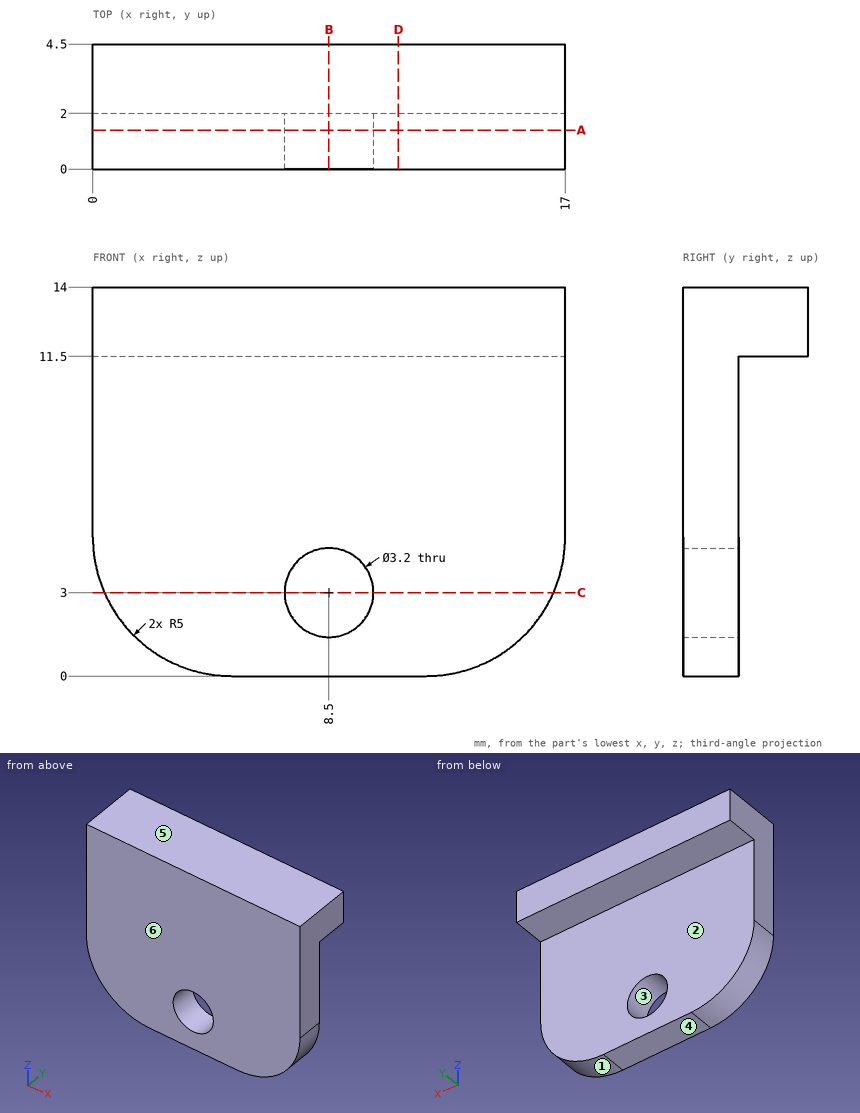
Geometry: see drawing. Coordinates: mm, zero at the bounding-box minimum. A direction names the side the tool comes from. Give positions to 0.01 mm unless a question says otherwise; leave off trailing zeros. Loops run counter-clockwise (first coordinate to the right, second up) from the corner with the lowest first, then second, coordinate; pieces in that order, holes last. Notation, with made-up numbers: (1.25, 31) - (52.25, 31) arc R16 ccw to (52.25, 42) - close; hole circle Ø1 at (65, -21.5). An arc over 180 degrees is marked (long way). Use CSV: the item, a comma, the result in double quotes. Start each with the question number.
Item 1: Mould query, pull axis Z, two halves, no side actions, for the marked faces 3, 4, 5 and 6. Classes: pulls with the +Z half, pulls with the -Z half, needs draft (parallel to the pull), parting line crosses it, or undercut.
Item 2: Section A-A on y = 1.4. Return loops of the section in (x, z).
Item 3: Line query: line 1 (Z direction, x = 8.5, y = 0.65); line 2 (Y direction, x = 1.5, z = 4.5); line 3 (Z direction, x = 13.25, y = 2.15). Output: solid intervals per line, ascending.
Item 4: Section C-C on z = 3. Return loops of the section in (x, y).
Item 5: Reachability of the marked faces 1 and 2 from +Z, -Z, +X, -X, +Y, -Y: full face, straight path, thin tool, end or side. Return the list, or none.
Item 6: Section B-B on x = 8.5. Return loops of the section in (y, z).
Item 7: Section D-D on x = 11. Return loops of the section in (y, z), then the cut area to 4 significant figures.
Item 8: Contact query for flat-ended pins moving along their axis: P1, Ø3, axis at x = 14.5, z = 10.5, coming from the +Y side; P2, Ø3, axis at x = 13.5, z = 2, coming from the +Y side; P3, Ø1.2, axis at x = 4.5, y = 3, coming from the -Z side. Output: stop coordinate, or through.
Ans:
1,face 3,"undercut"
1,face 4,"pulls with the -Z half"
1,face 5,"pulls with the +Z half"
1,face 6,"needs draft"
2,outline,"(0, 5) arc R5 ccw to (5, 0) - (12, 0) arc R5 ccw to (17, 5) - (17, 14) - (0, 14) - close; hole circle Ø3.2 at (8.5, 3)"
3,line 1,"z = 0 to 1.4, 4.6 to 14"
3,line 2,"y = 0 to 2"
3,line 3,"z = 11.5 to 14"
4,outline,"(0.42, 0) - (6.9, 0) - (6.9, 2) - (0.42, 2) - close; (10.1, 0) - (16.58, 0) - (16.58, 2) - (10.1, 2) - close"
5,face 1,"-Z, +X, +Y, -Y"
5,face 2,"-Z, +X, -X, +Y"
6,outline,"(0, 0) - (2, 0) - (2, 1.4) - (0, 1.4) - close; (0, 4.6) - (2, 4.6) - (2, 11.5) - (4.5, 11.5) - (4.5, 14) - (0, 14) - close"
7,outline,"(0, 0) - (2, 0) - (2, 11.5) - (4.5, 11.5) - (4.5, 14) - (0, 14) - close"
7,area,"34.25 mm2"
8,P1,"stops at y = 4.5"
8,P2,"stops at y = 2"
8,P3,"stops at z = 11.5"
